```python
from build123d import *

# Parameters (mm, degrees)
F0_W      = 76.2
F0_H      = 44.45
F1_DEPTH  = 10
F3_W      = 60.96
F3_H      = 35
F5_DEPTH  = 5
F6_DEPTH  = 3
F7_DEPTH  = 5
F8_DEPTH  = 3
F9_R      = 5.08
F10_W     = 3.1023733318
F10_H     = 3.9349872386
F11_DEPTH = 11
F12_W     = 42.3543415964
F12_H     = 1.6788681969
F13_DEPTH = 3
F4_R      = 0.5
F14_DEPTH = 8
F16_DEPTH = 3
F17_W     = 1.7839074135
F17_H     = 13.8109410182
F17_W_2   = 12.2273676097
F17_H_2   = 2.1280329674
F18_DEPTH = 3


with BuildPart() as f1:
    # F0 (on Top) → F1 (new body)
    with BuildSketch(Plane.XY):
        Rectangle(F0_W, F0_H)
        with BuildLine():
            Line((-30.0455586378, -5.2290757074), (-30.0455586378, 5.0972730335))
            ThreePointArc((-30.0455586378, 5.0972730335), (-30.1515789958, 14.6432590947), (-21.8663889779, 9.9006104081))
            ThreePointArc((-21.8663889779, 9.9006104081), (-22.9155259968, 6.6695395757), (-25.6626866956, 4.6711363874))
            Line((-25.6626866956, 4.6711363874), (-25.6626866956, 1.9259689143))
            Line((-25.6626866956, 1.9259689143), (26.3650547713, 1.9259689143))
            Line((26.3650547713, 1.9259689143), (28.737584129, 1.9259689143))
            Line((28.737584129, 1.9259689143), (28.737584129, -2.0090183243))
            Line((28.737584129, -2.0090183243), (26.3650547713, -2.0090183243))
            Line((26.3650547713, -2.0090183243), (-25.6626866956, -2.0090183243))
            Line((-25.6626866956, -2.0090183243), (-25.6626866956, -4.8029390612))
            ThreePointArc((-25.6626866956, -4.8029390612), (-22.9155259968, -6.8013422496), (-21.8663889779, -10.0324130819))
            ThreePointArc((-21.8663889779, -10.0324130819), (-30.1515789958, -14.7750617685), (-30.0455586378, -5.2290757074))
        make_face(mode=Mode.SUBTRACT)
    extrude(amount=F1_DEPTH)

    # F3 (on face) → F5 (cut)
    with BuildSketch(Plane.XY.offset(10)):
        with Locations((-4.8115077713, -2.409234643)):
            Rectangle(F3_W, F3_H)
    extrude(amount=-F5_DEPTH, mode=Mode.SUBTRACT)

    # F0 (on Top) → F6 (cut)
    with BuildSketch(Plane.XY):
        with BuildLine():
            ThreePointArc((-30.0455586378, 5.0972730335), (-28.7505212765, 4.5776246125), (-27.3663889779, 4.4006104081))
            ThreePointArc((-27.3663889779, 4.4006104081), (-26.5038656779, 4.468662916), (-25.6626866956, 4.6711363874))
            ThreePointArc((-25.6626866956, 4.6711363874), (-22.9155259968, 6.6695395757), (-21.8663889779, 9.9006104081))
            ThreePointArc((-21.8663889779, 9.9006104081), (-30.1515789958, 14.6432590947), (-30.0455586378, 5.0972730335))
        make_face()
        with BuildLine():
            ThreePointArc((-25.6626866956, -4.8029390612), (-26.5038656779, -4.6004655898), (-27.3663889779, -4.5324130819))
            ThreePointArc((-27.3663889779, -4.5324130819), (-28.7505212765, -4.7094272864), (-30.0455586378, -5.2290757074))
            ThreePointArc((-30.0455586378, -5.2290757074), (-30.1515789958, -14.7750617685), (-21.8663889779, -10.0324130819))
            ThreePointArc((-21.8663889779, -10.0324130819), (-22.9155259968, -6.8013422496), (-25.6626866956, -4.8029390612))
        make_face()
    extrude(amount=F6_DEPTH, mode=Mode.SUBTRACT)

    # F0 (on Top) → F7 (join)
    with BuildSketch(Plane.XY):
        Polygon((26.3650547713, 1.9259689143), (-25.6626866956, 1.9259689143), (-25.6626866956, -2.0090183243), (26.3650547713, -2.0090183243), (28.737584129, -2.0090183243), (28.737584129, 1.9259689143), align=None)
        with BuildLine():
            ThreePointArc((-25.6626866956, -4.8029390612), (-26.5038656779, -4.6004655898), (-27.3663889779, -4.5324130819))
            ThreePointArc((-27.3663889779, -4.5324130819), (-28.7505212765, -4.7094272864), (-30.0455586378, -5.2290757074))
            ThreePointArc((-30.0455586378, -5.2290757074), (-30.1515789958, -14.7750617685), (-21.8663889779, -10.0324130819))
            ThreePointArc((-21.8663889779, -10.0324130819), (-22.9155259968, -6.8013422496), (-25.6626866956, -4.8029390612))
        make_face()
        with BuildLine():
            Line((-27.3663889779, -4.5324130819), (-27.3663889779, 4.4006104081))
            ThreePointArc((-27.3663889779, 4.4006104081), (-28.7505212765, 4.5776246125), (-30.0455586378, 5.0972730335))
            Line((-30.0455586378, 5.0972730335), (-30.0455586378, -5.2290757074))
            ThreePointArc((-30.0455586378, -5.2290757074), (-28.7505212765, -4.7094272864), (-27.3663889779, -4.5324130819))
        make_face()
        with BuildLine():
            ThreePointArc((-30.0455586378, 5.0972730335), (-28.7505212765, 4.5776246125), (-27.3663889779, 4.4006104081))
            ThreePointArc((-27.3663889779, 4.4006104081), (-26.5038656779, 4.468662916), (-25.6626866956, 4.6711363874))
            ThreePointArc((-25.6626866956, 4.6711363874), (-22.9155259968, 6.6695395757), (-21.8663889779, 9.9006104081))
            ThreePointArc((-21.8663889779, 9.9006104081), (-30.1515789958, 14.6432590947), (-30.0455586378, 5.0972730335))
        make_face()
        with BuildLine():
            ThreePointArc((-25.6626866956, 4.6711363874), (-26.5038656779, 4.468662916), (-27.3663889779, 4.4006104081))
            Line((-27.3663889779, 4.4006104081), (-27.3663889779, -4.5324130819))
            ThreePointArc((-27.3663889779, -4.5324130819), (-26.5038656779, -4.6004655898), (-25.6626866956, -4.8029390612))
            Line((-25.6626866956, -4.8029390612), (-25.6626866956, -2.0090183243))
            Line((-25.6626866956, -2.0090183243), (-25.6626866956, 1.9259689143))
            Line((-25.6626866956, 1.9259689143), (-25.6626866956, 4.6711363874))
        make_face()
    extrude(amount=F7_DEPTH)

    # F0 (on Top) → F8 (cut)
    with BuildSketch(Plane.XY):
        Polygon((26.3650547713, 1.9259689143), (-25.6626866956, 1.9259689143), (-25.6626866956, -2.0090183243), (26.3650547713, -2.0090183243), (28.737584129, -2.0090183243), (28.737584129, 1.9259689143), align=None)
        with BuildLine():
            ThreePointArc((-30.0455586378, 5.0972730335), (-28.7505212765, 4.5776246125), (-27.3663889779, 4.4006104081))
            ThreePointArc((-27.3663889779, 4.4006104081), (-26.5038656779, 4.468662916), (-25.6626866956, 4.6711363874))
            ThreePointArc((-25.6626866956, 4.6711363874), (-22.9155259968, 6.6695395757), (-21.8663889779, 9.9006104081))
            ThreePointArc((-21.8663889779, 9.9006104081), (-30.1515789958, 14.6432590947), (-30.0455586378, 5.0972730335))
        make_face()
        with BuildLine():
            Line((-27.3663889779, -4.5324130819), (-27.3663889779, 4.4006104081))
            ThreePointArc((-27.3663889779, 4.4006104081), (-28.7505212765, 4.5776246125), (-30.0455586378, 5.0972730335))
            Line((-30.0455586378, 5.0972730335), (-30.0455586378, -5.2290757074))
            ThreePointArc((-30.0455586378, -5.2290757074), (-28.7505212765, -4.7094272864), (-27.3663889779, -4.5324130819))
        make_face()
        with BuildLine():
            ThreePointArc((-25.6626866956, 4.6711363874), (-26.5038656779, 4.468662916), (-27.3663889779, 4.4006104081))
            Line((-27.3663889779, 4.4006104081), (-27.3663889779, -4.5324130819))
            ThreePointArc((-27.3663889779, -4.5324130819), (-26.5038656779, -4.6004655898), (-25.6626866956, -4.8029390612))
            Line((-25.6626866956, -4.8029390612), (-25.6626866956, -2.0090183243))
            Line((-25.6626866956, -2.0090183243), (-25.6626866956, 1.9259689143))
            Line((-25.6626866956, 1.9259689143), (-25.6626866956, 4.6711363874))
        make_face()
        with BuildLine():
            ThreePointArc((-25.6626866956, -4.8029390612), (-26.5038656779, -4.6004655898), (-27.3663889779, -4.5324130819))
            ThreePointArc((-27.3663889779, -4.5324130819), (-28.7505212765, -4.7094272864), (-30.0455586378, -5.2290757074))
            ThreePointArc((-30.0455586378, -5.2290757074), (-30.1515789958, -14.7750617685), (-21.8663889779, -10.0324130819))
            ThreePointArc((-21.8663889779, -10.0324130819), (-22.9155259968, -6.8013422496), (-25.6626866956, -4.8029390612))
        make_face()
    extrude(amount=F8_DEPTH, mode=Mode.SUBTRACT)

    # F9
    f9_edges = [f1.edges().sort_by_distance(p)[0] for p in [
        (38.1, 22.225, 5),
        (38.1, -22.225, 5),
        (-38.1, -22.225, 5),
        (-38.1, 22.225, 5),
    ]]
    fillet(f9_edges, radius=F9_R)

    # F10 (on face) → F11 (cut)
    with BuildSketch(Plane.XY.offset(10)):
        with Locations((27.1863974631, -0.041524705)):
            Rectangle(F10_W, F10_H)
    extrude(amount=-F11_DEPTH, mode=Mode.SUBTRACT)

    # F12 (on face) → F13 (cut)
    with BuildSketch(Plane.XY):
        with Locations((-0.0403206795, -14.995015692)):
            Rectangle(F12_W, F12_H)
        with Locations((-0.0403206795, 14.995015692)):
            Rectangle(F12_W, F12_H)
    extrude(amount=F13_DEPTH, mode=Mode.SUBTRACT)

    # F4 (on face) → F14 (cut)
    with BuildSketch(Plane.XY.offset(10)):
        with Locations((-14.7766097486, 17.6294427365)):
            Circle(F4_R)
        with BuildLine():
            Line((30.7233902514, 17.6294427365), (31.2233902514, 17.6294427365))
            Line((31.2233902514, 17.6294427365), (31.2233902514, 17.1294427365))
            ThreePointArc((31.2233902514, 17.1294427365), (31.576943642, 17.2758893459), (31.7233902514, 17.6294427365))
            ThreePointArc((31.7233902514, 17.6294427365), (31.2233902514, 18.1294427365), (30.7233902514, 17.6294427365))
        make_face()
        with BuildLine():
            ThreePointArc((31.7233902514, 0.6294427365), (31.576943642, 0.9829961271), (31.2233902514, 1.1294427365))
            ThreePointArc((31.2233902514, 1.1294427365), (30.8698368608, 0.2758893459), (31.7233902514, 0.6294427365))
        make_face()
    extrude(amount=-F14_DEPTH, mode=Mode.SUBTRACT)

    # F15 (on face) → F16 (cut)
    with BuildSketch(Plane.XY):
        with BuildLine():
            Line((32.6728916039, -1.6812667771), (37.7627563252, -1.6541663098))
            ThreePointArc((37.7627563252, -1.6541663098), (37.9645099731, -1.5929708523), (38.1, -1.4314410684))
            Line((38.1, -1.4314410684), (38.1, 1.4314410684))
            ThreePointArc((38.1, 1.4314410684), (37.9645099731, 1.5929708523), (37.7627563252, 1.6541663098))
            Line((37.7627563252, 1.6541663098), (32.6728916039, 1.6812667771))
            ThreePointArc((32.6728916039, 1.6812667771), (32.4101390596, 1.5736086497), (32.3012533523, 1.3113624396))
            Line((32.3012533523, 1.3113624396), (32.3021029201, 0))
            Line((32.3021029201, 0), (32.3012533523, -1.3113624396))
            ThreePointArc((32.3012533523, -1.3113624396), (32.4101390596, -1.5736086497), (32.6728916039, -1.6812667771))
        make_face()
    extrude(amount=F16_DEPTH, mode=Mode.SUBTRACT)

    # F17 (on face) → F18 (cut)
    with BuildSketch(Plane.XY.offset(10)):
        with Locations((31.2101058662, -10.862109717)):
            Rectangle(F17_W, F17_H)
        with Locations((-27.7256574482, 19.1172780469)):
            Rectangle(F17_W_2, F17_H_2)
    extrude(amount=-F18_DEPTH, mode=Mode.SUBTRACT)


solid = f1.part
```
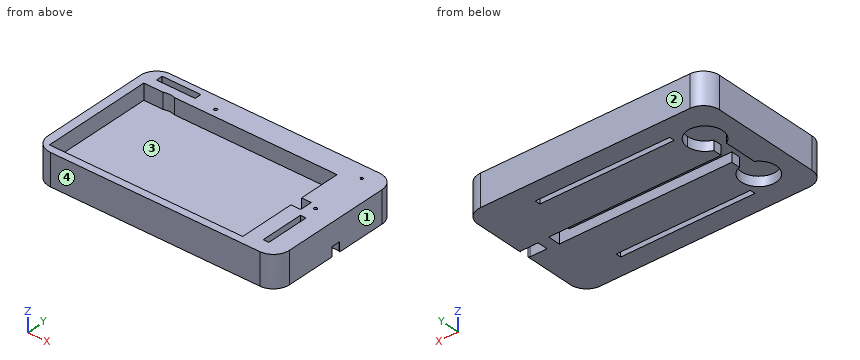
Geometry check sheet. Reference: the model listing, model coordinates, mm. Face numbers are marked on the shaded views. Coordinates: 2 decimals unless noted, no trailing zeros. Order: outer loops, then holes, each group sorted by start corner. A loop starts at its lowest first (then second) coordinate and runs counter-clockwise, first axis right, second up.
Q1. Draft check along Y on the marked faces 1, 2, 3 and 4. Enter one of: released by +Y, released by -Y, zero draft, split by the parting line, or undercut.
Reply:
face 1: zero draft
face 2: released by +Y
face 3: undercut
face 4: released by -Y
Q2. Depth check by flat-ended pin: pin 1 Ø6 at (x, y) = (-7, -6) entering from +Z; pin 2 Ø1.7 at (y, z) = (18.5, 8.5) entering from +X; pin 3 Ø10 at (x, y) = (-27.37, -10.03) entering from -Z. Enter the tip coordinate at first touch or a pass-through.
Reply:
pin 1: stops at z = 5
pin 2: stops at x = 38.07
pin 3: stops at z = 3
Q3. Sectioned sample at B-B on x = -18. Record the cut outline in (y, z) (3 decimals), and give its area (3 significant figures).
Reply:
outline: (-22.225, 0) - (-15.834, 0) - (-15.834, 3) - (-14.156, 3) - (-14.156, 0) - (-2.009, 0) - (-2.009, 3) - (1.926, 3) - (1.926, 0) - (14.156, 0) - (14.156, 3) - (15.834, 3) - (15.834, 0) - (22.225, 0) - (22.225, 10) - (15.091, 10) - (15.091, 5) - (-19.909, 5) - (-19.909, 10) - (-22.225, 10) - close
area: 248 mm2
Q4. Thickness scan on probe 1 along Y at (x, z) = (-6, 2) (3 decimals); probe 2 along Y at (x, z) = (-22.5, 7.25) (3 decimals); probe 3 along X at (y, z) = (-14, 8). Record the ranges inside material, lowest first.
Reply:
probe 1: y = -22.225 to -15.834, -14.156 to -2.009, 1.926 to 14.156, 15.834 to 22.225
probe 2: y = -22.225 to -19.909, 15.091 to 18.053, 20.181 to 22.225
probe 3: x = -38.1 to -35.29, 25.67 to 30.32, 32.1 to 38.1
Q5. Sectioned sample at D-D on y = -7. Record the cut outline in (x, z).
Reply:
outline: (-38.1, 0) - (-31.95, 0) - (-31.95, 3) - (-22.78, 3) - (-22.78, 0) - (38.1, 0) - (38.1, 10) - (32.1, 10) - (32.1, 7) - (30.32, 7) - (30.32, 10) - (25.67, 10) - (25.67, 5) - (-35.29, 5) - (-35.29, 10) - (-38.1, 10) - close
Q6. Sectioned sample at A-A on z = 1.25. Give the number of separate pieces and of enclosed holes in the cut face, and give its area (3 significant figures).
Reply:
separate pieces: 1
enclosed holes: 3
area: 2,760 mm2
